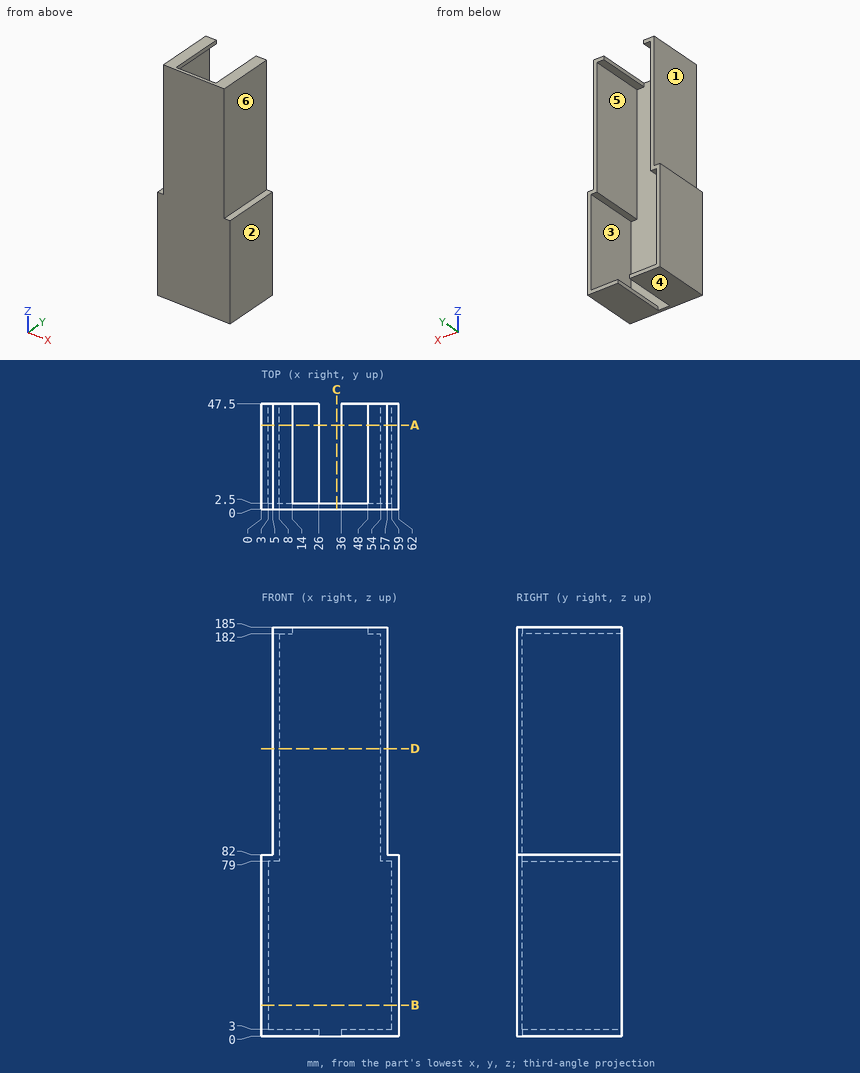
Input: dimensioned drawing with shaded views. Units: mm. Origin: part minimum x, y, z. A direction names the side the tool comes from. Round coordinates to 2 decimals unless told otherwise and drop trailing zeros. Loops run counter-clockwise (first coordinate to the right, second up) from the corner with the lowest first, then second, coordinate; pieces in that order, holes last. Notation, with made-up numbers: (7.25, 79) -> (28.25, 79) arc R21 cw to (28.25, 87) -> close; hole circle Ø5 at (35, 73.5). An arc over 180 degrees is marked (long way). Answer as a JSON object with one key per item and string values. Group by question number.
1) Reachability of the marked faces 1, 2 and 3 from +Z, -Z, +X, -X, +Y, -Y: full face, straight path, thin tool, end or side. Return the list, or none.
2) Section query A-A on y = 38. Output: boundary loops of the cut face in (x, z).
3) Section query D-D on z = 130. Output: boundary loops of the cut face in (x, y).
4) Draft query along Z for the marked faces 4, 5 and 6. Return one class per face: +Z half, -Z half, draft (parallel to the pull), parting line (faces both ways), or undercut.
5) Ray query, L1, parallel to X at y = 31, z = 151; L2, parallel to X at y = 29, z = 75.5; L3, parallel to Z at x = 53.5, y = 17. Return the intervals inside material, ascending.
6) Section query C-C on x = 34. Output: boundary loops of the cut face in (y, z), plus the area to 4 significant figures.
7) Section query B-B on z = 14. Output: boundary loops of the cut face in (x, y).
8) Pin query (flat end, axial travel): pin 1 (10 mm diameter, centred on x = 30.5, z = 149, fed in from +Y); pin 2 (6 mm diameter, centred on x = 40.5, y = 12, fed in from +Z); pin 3 (14 mm diameter, centred on y = 25, z = 155.5, fed in from +X). Return the tip coordinate at first contact, or that it passes through.
Reply:
{
 "1": {"face 1": "+Z, -X, +Y, -Y", "face 2": "+Z, -Z, +X, +Y, -Y", "face 3": "+Y"},
 "2": {"outline": "(0, 0) -> (26, 0) -> (26, 3) -> (3, 3) -> (3, 79) -> (8, 79) -> (8, 182) -> (14, 182) -> (14, 185) -> (5, 185) -> (5, 82) -> (0, 82) -> close; (36, 0) -> (62, 0) -> (62, 82) -> (57, 82) -> (57, 185) -> (48, 185) -> (48, 182) -> (54, 182) -> (54, 79) -> (59, 79) -> (59, 3) -> (36, 3) -> close"},
 "3": {"outline": "(5, 0) -> (57, 0) -> (57, 47.5) -> (54, 47.5) -> (54, 2.5) -> (8, 2.5) -> (8, 47.5) -> (5, 47.5) -> close"},
 "4": {"face 4": "-Z half", "face 5": "undercut", "face 6": "draft"},
 "5": {"L1": "x = 5 to 8, 54 to 57", "L2": "x = 0 to 3, 59 to 62", "L3": "z = 0 to 3, 182 to 185"},
 "6": {"outline": "(0, 0) -> (2.5, 0) -> (2.5, 185) -> (0, 185) -> close", "area": "462.5 mm2"},
 "7": {"outline": "(0, 0) -> (62, 0) -> (62, 47.5) -> (59, 47.5) -> (59, 2.5) -> (3, 2.5) -> (3, 47.5) -> (0, 47.5) -> close"},
 "8": {"pin 1": "stops at y = 2.5", "pin 2": "stops at z = 3", "pin 3": "stops at x = 57"}
}
